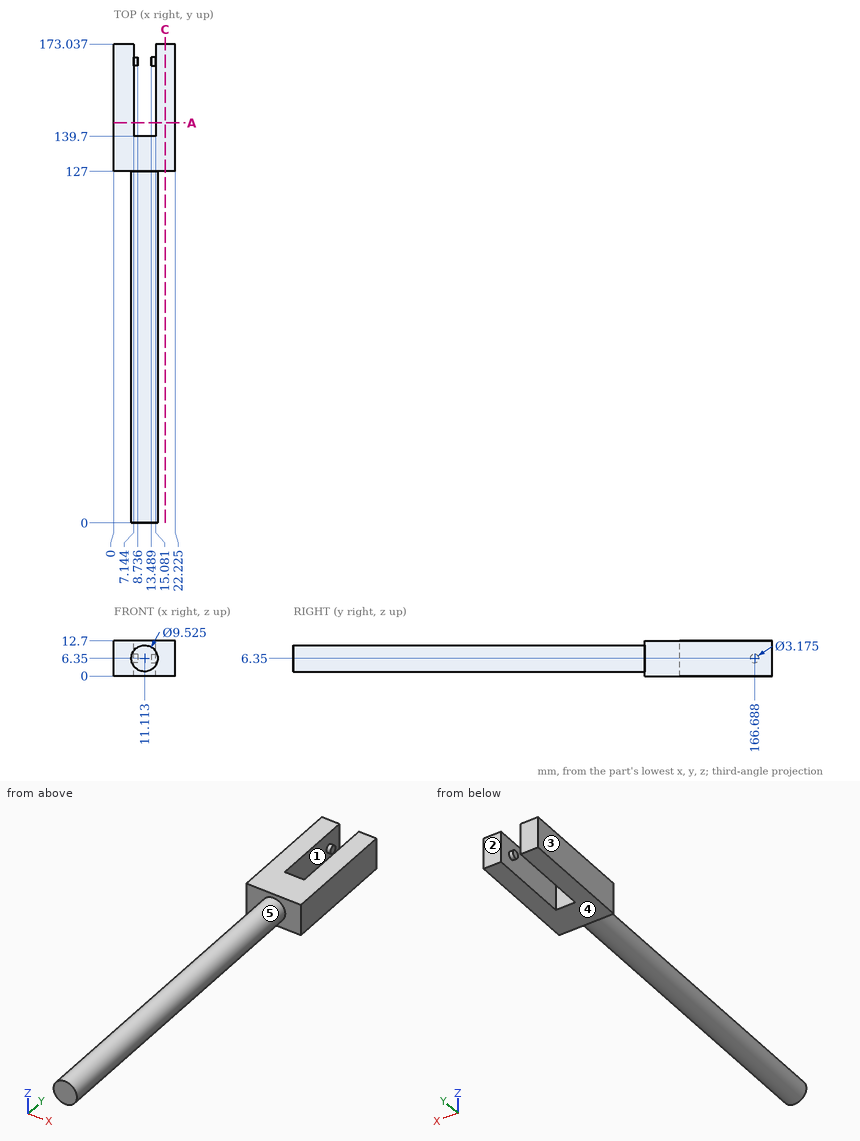
Answer from the drawing. Dimensions are ordinates in mm from the lowest x, y and z of the part. A direction names the side the tool comes from. Give positions to 0.01 mm unless a question says otherwise; leave off trailing zeros. Write each loop counter-clockwise with the first axis right and the second up, starting at its lowest first coordinate (ties: lowest second). Pieces come first, ordered by that corner, then holes. Notation, with made-up numbers: (13.5, 55) -> (43.5, 55) arc R19 ccw to (43.5, 61) -> close; hole circle Ø11 at (43, 47). An arc over 180 degrees is marked (long way). One line per question, with ' | ' between items. Start each with the question number.
1. Find the intervals of material crossed by probe 1 along X at (y, z) = (152, 6.75) (1 decimal); probe 2 along Y at (x, z) = (15, 10); probe 3 along Z at (x, y) = (11, 51), in increasing order.
2. For the marked faces 4 and 5, determine the directions among +Z, -Z, +X, -X, +Y, -Y from which every point of the face is accessible in a straight line to the end or side of a thin tool.
3. For a pull along X with two mould halves and no side action, classify the marked faces 1, 2 and 3 as pulls with the +X half, pulls with the -X half, needs draft (parallel to the pull), parting line crosses it, or undercut.
4. Section A-A (y = 144.5) is taken. Determine the outline of the cut face in (x, z) (1 decimal).
5. Section C-C (x = 18.5) is taken. Determine the outline of the cut face in (y, z), plus the area to 3 significant figures.
6. Given pin 1 Ø12 at (x, y) = (20, 91) entering from +Z; pin 2 Ø10 at (x, y) = (17, 64.5) entering from +Z; pin 3 Ø5 at (x, z) = (19.5, 6) entering from -Y, each flat-ended and moving along its own axis, determine where each tip first touches the part or whether it passes through.
Response values:
1) probe 1: 0 to 7.1, 15.1 to 22.2 | probe 2: 127 to 139.7 | probe 3: 1.59 to 11.11
2) face 4: -Z, +X, -X, +Y, -Y | face 5: -Y
3) face 1: undercut | face 2: needs draft | face 3: pulls with the -X half
4) outline: (0, 0) -> (7.1, 0) -> (7.1, 12.7) -> (0, 12.7) -> close; (15.1, 0) -> (22.2, 0) -> (22.2, 12.7) -> (15.1, 12.7) -> close
5) outline: (127, 0) -> (173.04, 0) -> (173.04, 12.7) -> (127, 12.7) -> close | area: 585 mm2
6) pin 1: z = 10.14 | pin 2: z = 11.03 | pin 3: y = 127
